Can you work these out from the model? Positions are in its coordinate system, mm. Give positions to 0.01 mm unless a question says otherwise; leave off trailing zeros. Loops run counter-clockwise (first coordinate to the right, second up) from the corner with the lowest first, then second, coordinate; pieces in that order, holes last. Notation, with made-up numbers: (21.25, 57.25) -> (38.25, 57.25) arc R22 ccw to (38.25, 96.25) -> close; hole circle Ø8 at (-18.5, 4.25). An arc over 180 degrees is marked (long way). Use CSV: the item, a comma, the result in double quotes.
from build123d import *

# Parameters (mm, degrees)
SKETCH1_W           = 106
SKETCH1_H           = 5
BOSS_EXTRUDE1_DEPTH = 5
FILLET1_R           = 1
FILLET2_R           = 1
SKETCH2_R           = 1
CUT_EXTRUDE1_DEPTH  = 54.293995909


with BuildPart() as part:
    # Sketch1 → Boss-Extrude1 (new body)
    with BuildSketch(Plane(origin=(0, 0, 0), x_dir=(1, 0, 0), z_dir=(0, 1, 0))):
        Rectangle(SKETCH1_W, SKETCH1_H)
    extrude(amount=BOSS_EXTRUDE1_DEPTH)

    # Fillet1
    fillet1_edges = [part.edges().sort_by_distance(p)[0] for p in [
        (-53, 2.5, 2.5),
        (-53, 2.5, -2.5),
    ]]
    fillet(fillet1_edges, radius=FILLET1_R)

    # Fillet2
    fillet2_edges = [part.edges().sort_by_distance(p)[0] for p in [
        (53, 2.5, 2.5),
        (53, 2.5, -2.5),
    ]]
    fillet(fillet2_edges, radius=FILLET2_R)

    # Sketch2 → Cut-Extrude1 (cut, through all)
    with BuildSketch(Plane(origin=(0, 5, 0), x_dir=(1, 0, 0), z_dir=(0, 1, 0))):
        with Locations(Location((-50, 0, 0), (0, 0, 270))):
            Circle(SKETCH2_R)
        with Locations(Location((50, 0, 0), (0, 0, 270))):
            Circle(SKETCH2_R)
        with Locations(Location((-2.5, 0, 0), (0, 0, 270))):
            Circle(SKETCH2_R)
        with Locations(Location((2.5, 0, 0), (0, 0, 270))):
            Circle(SKETCH2_R)
    extrude(amount=-CUT_EXTRUDE1_DEPTH, mode=Mode.SUBTRACT)


solid = part.part
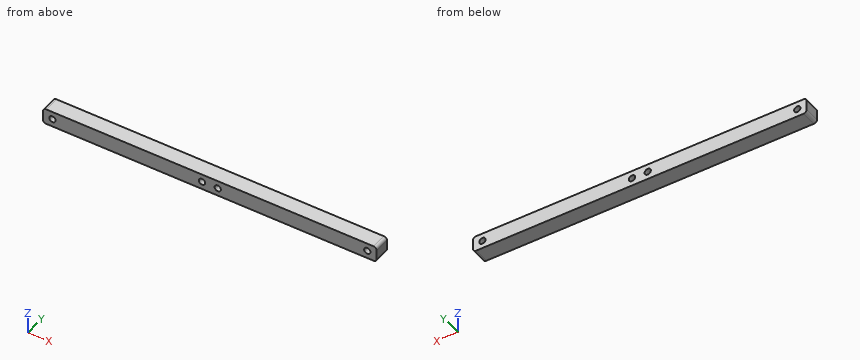
(1) Will this pin go through, and if not, where does the flat tip stop? pin 1 Ø1.8 at (x, z) = (50, 0) entering from -Y.
Answer sheet:
pin 1,"passes through"
(2) If I drill on L1, parallel to X at y = 1.2, z = -0.05; L2, parallel to X at y = 0.35, z = 0.6; L3, parallel to X at y = 0.3, z = -1.95, over which ranges is the centre line in solid material (lowest first)? Write a range as from..to.
Answer sheet:
L1,"x = -53..-51, -49..-3.5, -1.5..1.5, 3.5..49, 51..53"
L2,"x = -53..-50.8, -49.2..-3.3, -1.7..1.7, 3.3..49.2, 50.8..53"
L3,"x = -52.89..52.89"
(3) If we section it at A-A, the plane y = 2.2: Write out the boundary of the cut face in (x, z).
Answer sheet:
outline,"(-53, -1.5) arc R1 ccw to (-52, -2.5) -> (52, -2.5) arc R1 ccw to (53, -1.5) -> (53, 1.5) arc R1 ccw to (52, 2.5) -> (-52, 2.5) arc R1 ccw to (-53, 1.5) -> close; hole circle Ø2 at (-50, 0); hole circle Ø2 at (-2.5, 0); hole circle Ø2 at (2.5, 0); hole circle Ø2 at (50, 0)"
(4) If we section it at B-B, the plane x = 2.5: Write out the boundary of the cut face in (y, z), then the cut area to 3 significant figures.
Answer sheet:
outline,"(0, -2.5) -> (5, -2.5) -> (5, -1) -> (0, -1) -> close; (0, 1) -> (5, 1) -> (5, 2.5) -> (0, 2.5) -> close"
area,"15.0 mm2"
